Autodesk Inventor part; units mm, degrees
ref_plane "Plano de trabajo1" through (-95, 0, 0) normal (0, 0, -1) x (-1, 0, 0)
ref_plane "YZ Plane" through (0, 0, 0) normal (1, 0, 0) x (0, 1, 0)
ref_plane "XZ Plane" through (0, 0, 0) normal (0, 1, 0) x (-1, 0, 0)
sketch "Boceto2" plane through (0, 0, 0) normal (0, 0, 1) x (1, 0, 0)
  line L0 (130, -85) -> (-130, -85)
  line L1 (-130, -85) -> (-130, 85)
  line L2 (-130, 85) -> (130, 85)
  line L3 (130, 85) -> (130, -85)
  line L4 (130, -85) -> (-130, 85) construction
  line L5 (-130, -85) -> (130, 85) construction
  point P0 (0, 0)
  dimension "d0" = 260
  dimension "d1" = 170
extrude "Extrusión1" add sketch "Boceto2" along normal blind 5
sketch "Boceto3" plane through (0, 0, 5) normal (0, 0, 1) x (1, 0, 0)
  line L0 (-95, 0) -> (-4.19, 0) construction
  circle A0 centre (-95, 0) radius 2.625
  circle A1 centre (-4.19, 0) radius 9.875
  line L1 (-130, 85) -> (-130, -85)
  line L2 (130, -85) -> (130, 85)
  line L3 (-130, -85) -> (130, -85)
  line L4 (130, 0) -> (80, 0) construction
  line L5 (80, 0) -> (80, -23.2237) construction
  arc A2 (-110, -17.625) -> (-110, 17.625) centre (-110, 0) ccw
  arc A3 (-110, -12.375) -> (-110, 12.375) centre (-110, 0) ccw
  arc A4 (-110, 17.625) -> (-110, 12.375) centre (-110, 15) ccw
  arc A5 (-110, -12.375) -> (-110, -17.625) centre (-110, -15) ccw
  point P0 (0, 0)
  point P1 (-130, 0)
  point P2 (-92.375, 0)
  point P3 (-97.625, 0)
  dimension "d7" = 5.25
  dimension "d8" = 19.75
  dimension "d14" = 85
  dimension "d29" = 50
  dimension "d31" = 35
  dimension "d32" = 134.19
sketch "Boceto5" plane through (0, 0, 0) normal (0, 0, -1) x (-1, 0, 0)
  line L0 (-130, -85) -> (-130, 85)
  line L1 (130, -85) -> (-130, -85)
  line L2 (-130, -85) -> (-130, 85)
  line L3 (-130, 85) -> (130, 85)
  line L4 (130, 85) -> (130, -85)
  line L5 (130, -85) -> (-130, 85) construction
  line L6 (-130, -85) -> (130, 85) construction
  line L7 (119.5, 74.5) -> (-119.5, 74.5)
  line L8 (-119.5, 74.5) -> (-119.5, -74.5)
  line L9 (-119.5, -74.5) -> (119.5, -74.5)
  line L10 (119.5, -74.5) -> (119.5, 74.5)
  circle A0 centre (95, 0) radius 2.625
  circle A1 centre (95, 0) radius 2.625
  point P0 (0, 0)
  dimension "d23" = 10.5
  dimension "d25" = 5.25
extrude "Extrusión4" [suppressed]
sketch "Boceto6" plane through (0, 0, 5) normal (0, 0, 1) x (1, 0, 0)
  circle A0 centre (-4.19, 0) radius 10.125
  line L0 (-4.19, 0) -> (35.81, 0)
  line L1 (35.81, 0) -> (35.81, 25)
  line L2 (37.81, 23.5) -> (33.81, 23.5)
  line L3 (33.81, 23.5) -> (33.81, 26.5)
  line L4 (33.81, 26.5) -> (37.81, 26.5)
  line L5 (37.81, 26.5) -> (37.81, 23.5)
  line L6 (37.81, 23.5) -> (33.81, 26.5) construction
  line L7 (33.81, 23.5) -> (37.81, 26.5) construction
  point P0 (0, 0)
  dimension "d35" = 40
  dimension "d36" = 25
  dimension "d38" = 4
  dimension "d39" = 3
extrude "Extrusión5" cut sketch "Boceto6" against normal blind 1.4 contours L2 L3 L4 L5
sketch "Boceto8" plane through (0, 0, 5) normal (0, 0, 1) x (1, 0, 0)
  line L0 (33.81, 23.5) -> (33.81, 26.5)
  line L1 (33.81, 23.5) -> (37.81, 23.5)
  line L2 (37.81, 23.5) -> (37.81, 22.5)
  line L3 (37.81, 22.5) -> (33.81, 22.5)
  line L4 (33.81, 22.5) -> (33.81, 23.5)
  point P0 (0, 0)
  dimension "d42" = 4
  dimension "d43" = 1
extrude "Extrusión6" cut sketch "Boceto8" against normal through all
sketch "Boceto10" plane through (0, 0, -4) normal (0, 0, -1) x (-1, 0, 0)
  circle A0 centre (95, 0) radius 2.625
  circle A1 centre (95, 0) radius 7.5
  point P0 (0, 0)
  dimension "d51" = 15
ref_plane "Plano de trabajo1" through (-95, 0, 0) normal (0, 0, -1) x (-1, 0, 0)
sketch "Boceto12" plane through (0, 0, 5) normal (0, 0, 1) x (1, 0, 0)
  circle A0 centre (-95, 0) radius 2.625 construction
  circle A1 centre (-95, 0) radius 18.5 construction
  circle A2 centre (-95, 0) radius 20 construction
  circle A3 centre (-95, 0) radius 7.5 construction
  line L0 (-95, 0) -> (-82.5, 0) construction
  circle A4 centre (-82.5, 0) radius 3
  line L1 (-95, 0) -> (-107.5, 0) construction
  circle A5 centre (-107.5, 0) radius 3
  circle A6 centre (-107.5, 0) radius 1.5 construction
  circle A7 centre (-82.5, 0) radius 1.5 construction
  line L2 (-82.5, 0) -> (-97.5, 0) construction
  line L3 (-97.5, 0) -> (-97.5, 18.5) construction
  arc A8 (-89.1168, -15.9286) -> (-89.9998, 16.363) centre (-97.5, 0) ccw
  arc A9 (-91.9112, -10.6191) -> (-92.6345, 10.9694) centre (-97.5, 0) ccw
  arc A10 (-91.9112, -10.6191) -> (-89.1168, -15.9286) centre (-90.514, -13.2739) ccw
  arc A11 (-89.9998, 16.363) -> (-92.6345, 10.9694) centre (-91.2508, 13.6338) ccw
  arc A12 (-91.9112, -10.6191) -> (-89.1168, -15.9286) centre (-90.514, -13.2739) ccw
  arc A13 (-92.595, 10.9517) -> (-92.4052, 10.8647) centre (-91.2508, 13.6338) ccw
  arc A14 (-91.9112, -10.6191) -> (-89.1168, -15.9286) centre (-90.514, -13.2739) ccw
  arc A15 (-89.8154, -14.6013) -> (-90.6248, 14.9994) centre (-97.5, 0) ccw
  arc A16 (-90.6248, 14.9994) -> (-91.9757, 12.318) centre (-91.2508, 13.6338) ccw
  arc A17 (-91.2126, -11.9465) -> (-91.9757, 12.318) centre (-97.5, 0) ccw
  arc A18 (-91.2126, -11.9465) -> (-89.8154, -14.6013) centre (-90.514, -13.2739) ccw
  circle A19 centre (-82.5, 0) radius 1.5
  line L4 (-130, 85) -> (-130, -85)
  line L5 (-130, -85) -> (130, -85)
  point P0 (0, 0)
  point P1 (-89.8154, -14.6013)
  point P2 (-91.2126, -11.9465)
  point P3 (-84.225, -2.4545)
  point P4 (-85.5, 0)
  point P5 (-79.5, 0)
  point P6 (-81.225, -2.7156)
  point P7 (-84.225, 2.4545)
  point P8 (-81.225, 2.7156)
  point P9 (-84, 0)
  point P10 (-81, 0)
  dimension "d57" = 37
  dimension "d58" = 40
  dimension "d59" = 15
  dimension "d60" = 12.5
  dimension "d61" = 6
  dimension "d62" = 12.5
  dimension "d63" = 6
  dimension "d64" = 3
  dimension "d65" = 3
  dimension "d126" = 15
  dimension "d127" = 6
  dimension "d128" = 6
  dimension "d129" = 1.5
  dimension "d130" = 1.5
  dimension "d135" = 3
  dimension "d137" = 38.7492
  dimension "d138" = 98.6338
extrude "Extrusión10" cut sketch "Boceto12" against normal blind 1.5 contours A4 A15 | A15 A19 A17 A4 | A4 A17 A19 A15 | A17 A4 | A19 | A5
sketch "Boceto13" plane through (-82.5, 0, 3.5) normal (0, 0, 1) x (1, 0, 0)
  circle A0 centre (0, 0) radius 1.5
  circle A1 centre (-25, 0) radius 3
  circle A2 centre (-25, 0) radius 1.5
  point P0 (82.5, 0)
  dimension "d68" = 3
  dimension "d69" = 3
extrude "Extrusión11" cut sketch "Boceto13" against normal through all contours A0 | A2
extrude "Extrusión12" [suppressed]
extrude "Extrusión13" add sketch "Boceto3" along normal blind 10 contours A1
sketch "Boceto15" plane through (-4.19, 0, 15) normal (0, 0, 1) x (1, 0, 0)
  circle A0 centre (0, 0) radius 5
  circle A1 centre (0, 0) radius 74 construction
  circle A2 centre (-90.81, 0) radius 2.625 construction
  circle A3 centre (-90.81, 0) radius 20 construction
  point P0 (4.19, 0)
  dimension "d77" = 10
  dimension "d80" = 148
  dimension "d82" = 40
extrude "Extrusión14" cut sketch "Boceto15" against normal through all
sketch "Boceto16" plane through (0, 0, -4) normal (0, 0, -1) x (-1, 0, 0)
  line L0 (119.5, 74.5) -> (-119.5, 74.5)
  line L1 (-119.5, 74.5) -> (119.5, 74.5)
  line L2 (119.5, 74.5) -> (119.5, -74.5)
  line L3 (119.5, -74.5) -> (-119.5, -74.5)
  line L4 (-119.5, -74.5) -> (-119.5, 74.5)
  line L5 (-114.5, 69.5) -> (114.5, 69.5)
  line L6 (114.5, 69.5) -> (114.5, -69.5)
  line L7 (114.5, -69.5) -> (-114.5, -69.5)
  line L8 (-114.5, -69.5) -> (-114.5, 69.5)
  point P0 (0, 0)
  dimension "d83" = 5
extrude "Extrusión15" [suppressed]
sketch "Boceto17" plane through (0, 0, 5) normal (0, 0, 1) x (1, 0, 0)
  circle A0 centre (-95, 0) radius 2.625 construction
  circle A1 centre (-4.19, 0) radius 5 construction
  circle A2 centre (-4.19, 0) radius 40
  circle A3 centre (-4.19, 0) radius 15
  point P0 (0, 0)
  dimension "d87" = 80
  dimension "d88" = 30
sketch "Boceto20" plane through (0, 0, 5) normal (0, 0, 1) x (1, 0, 0)
  line L0 (130, 85) -> (-130, 85)
  line L1 (130, -85) -> (130, 85)
  line L2 (130, 85) -> (220, 85)
  line L3 (220, 85) -> (220, -85)
  line L4 (220, -85) -> (130, -85)
  line L5 (130, -85) -> (130, 85)
  point P0 (0, 0)
  dimension "d115" = 90
extrude "Extrusión22" add sketch "Boceto20" against normal blind 5
extrude "Extrusión23" cut sketch "Boceto3" against normal through all contours A0
extrude "Extrusión24" cut sketch "Boceto3" against normal blind 5 contours A2 A5 A3 A0 | A0 A3 A4 A2
extrude "Extrusión25" cut sketch "Boceto12" against normal blind 1.5 contours A8 A10 A9 A4 A17 A18 A15 | A4 A15 A16 A17 A9 A11 A8
extrude "Extrusión26" cut sketch "Boceto12" against normal through all contours A15 A19 A17 A4 | A4 A17 A16 A15 | A15 A18 A17 A4 | A4 A17 A19 A15
properties part number "Lid"
For this review, take the finished solid that the model builds, in its own axes (mm). A direction names the side the tool comes from. Round coordinates to 2 decimals unless told otherwise and drop trailing zeros. Write each loop counter-clockwise with the first axis right and the second up, starting at its lowest first coordinate (ties: lowest second). Pieces come first, ordered by that corner, then holes. Notation, with made-up numbers: (65, 75.5) - (73, 75.5) arc R17 ccw to (73, 82.5) - close; hole circle Ø10 at (-40, 23). An arc over 180 degrees is marked (long way). Use CSV: the item, a comma, the result in double quotes.
1) Wall thickness on line 1 along Y through (x, z) = (-107.5, 4); line 2 along Y through (x, z) = (-4.19, 3.5); line 3 along Y through (x, z) = (-101, 2.25): over which ranges is each line inside the solid? List them lowest first. Write a range as from..to.
Conclusion:
line 1,"y = -85..-17.45, -12.12..-3, 3..12.12, 17.45..85"
line 2,"y = -85..-5, 5..85"
line 3,"y = -85..-15.15, -8.49..8.49, 15.15..85"
2) Clearance check with flat-ended pins moving along their axes: pin 1 Ø8 at (x, y) = (6, 14) entering from +Z; pin 2 Ø3.5 at (x, y) = (-107.5, 0) entering from +Z; pin 3 Ø2.5 at (x, y) = (36, 24.5) entering from +Z. State where each tip first meets the part, or that it passes through.
Conclusion:
pin 1,"stops at z = 5"
pin 2,"stops at z = 3.5"
pin 3,"stops at z = 3.6"
3) The part is to be moulded in two halves that separate along Y. For faces 1 (the flat face through (-9, 2, 15)), 2 (the flat face through (-109, -1, 3.5)), 3 (the cylindrical face through (-11.47, -6.67, 9.93)), say which applies: pulls with the +Y half, pulls with the -Y half, needs draft (parallel to the pull), parting line crosses it, or undercut.
Conclusion:
face 1,"needs draft"
face 2,"undercut"
face 3,"parting line crosses it"
4) Add section B-B on z = 8.25. Write out the cut boundary in (x, y) (3 decimals), and give its area (3 significant figures).
Conclusion:
outline,"circle Ø19.75 at (-4.19, 0); hole circle Ø10 at (-4.19, 0)"
area,"228 mm^2"
5) Add section C-C on y = 30. Write out the cut boundary in (x, z).
Conclusion:
outline,"(-130, 0) - (220, 0) - (220, 5) - (-130, 5) - close"
6) Add section A-A on x = -4.19. Write out the cut boundary in (y, z) (3 decimals), and give its area (4 significant figures).
Conclusion:
outline,"(-85, 0) - (-5, 0) - (-5, 15) - (-9.875, 15) - (-9.875, 5) - (-85, 5) - close; (5, 0) - (85, 0) - (85, 5) - (9.875, 5) - (9.875, 15) - (5, 15) - close"
area,"897.5 mm^2"
7) For faces 4 (the cylindrical face through (-79.5, 0.2, 4.3)), 5 (the flat face through (43, 1, 0)), 6 (the cylindrical face through (-84, 0, 2)), list the 3-axis set-ups (+Z, -Z, +X, -X, +Y, -Y) from which the entire face can be reached by the end or side of a thin tool; tool diameter is ignored.
Conclusion:
face 4,"+Z"
face 5,"-Z, +X, -X, +Y, -Y"
face 6,"+Z, -Z"
